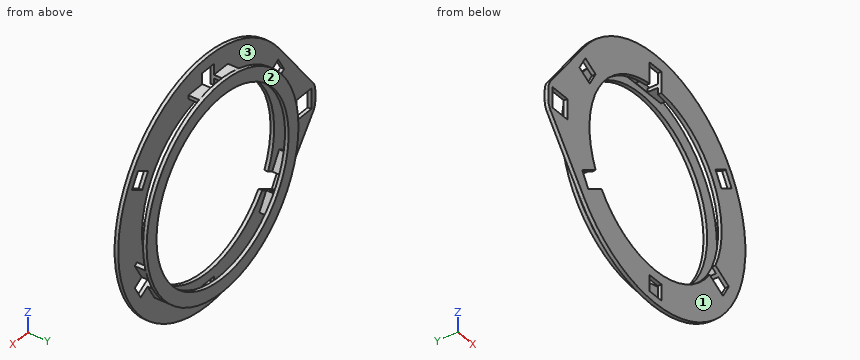
```python
from build123d import *

# Parameters (mm, degrees)
SKETCH1_R           = 340
SKETCH1_R_2         = 250
SKETCH1_W           = 44.45
SKETCH1_H           = 44.45
BOSS_EXTRUDE1_DEPTH = 10
BOSS_EXTRUDE2_DEPTH = 40
SKETCH3_W           = 44.45
SKETCH3_H           = 44.45
CUT_EXTRUDE1_DEPTH  = 30
CIRPATTERN1_COUNT   = 3
SKETCH4_R           = 287.263450512
SKETCH4_R_2         = 250
BOSS_EXTRUDE3_DEPTH = 10
BOSS_EXTRUDE4_DEPTH = 10
SKETCH6_W           = 57
SKETCH6_H           = 56.4
CUT_EXTRUDE2_DEPTH  = 10


with BuildPart() as part:
    # Sketch1 → Boss-Extrude1 (new body)
    with BuildSketch(Plane(origin=(0, 0, 0), x_dir=(1, 0, 0), z_dir=(0, 1, 0))):
        Circle(SKETCH1_R)
        Circle(SKETCH1_R_2, mode=Mode.SUBTRACT)
        with Locations((0, 297.225)):
            Rectangle(SKETCH1_W, SKETCH1_H, mode=Mode.SUBTRACT)
        Polygon((287.764315239, -140.477585401), (249.269486041, -118.252585401), (227.044486041, -156.747414599), (265.539315239, -178.972414599), align=None, mode=Mode.SUBTRACT)
        Polygon((-265.539315239, -178.972414599), (-227.044486041, -156.747414599), (-249.269486041, -118.252585401), (-287.764315239, -140.477585401), align=None, mode=Mode.SUBTRACT)
    extrude(amount=BOSS_EXTRUDE1_DEPTH)

    # Sketch2 → Boss-Extrude2 (add)
    with BuildSketch(Plane(origin=(0, 10, 0), x_dir=(1, 0, 0), z_dir=(0, 1, 0))):
        Polygon((22.25, -267.3), (-22.25, -267.3), (-75, -267.3), (-75, -277.3), (-22.25, -277.3), (22.25, -277.3), (75, -277.3), (75, -267.3), align=None)
        Polygon((-229.023844469, 157.919065234), (-202.648844469, 203.601905284), (-193.988590432, 198.601905284), (-220.363590432, 152.919065234), (-242.613590432, 114.380934766), (-268.988590432, 68.698094716), (-277.648844469, 73.698094716), (-251.273844469, 119.380934766), align=None)
        Polygon((251.273844469, 119.380934766), (277.648844469, 73.698094716), (268.988590432, 68.698094716), (242.613590432, 114.380934766), (220.363590432, 152.919065234), (193.988590432, 198.601905284), (202.648844469, 203.601905284), (229.023844469, 157.919065234), align=None)
    extrude(amount=BOSS_EXTRUDE2_DEPTH)

    # Sketch3 → Cut-Extrude1 (cut, symmetric)
    with BuildSketch(Plane.XY.offset(277.3)):
        with Locations((0, 16.699086593)):
            Rectangle(SKETCH3_W, SKETCH3_H)
    cut_extrude1 = extrude(amount=CUT_EXTRUDE1_DEPTH, both=True, mode=Mode.SUBTRACT)

    # CirPattern1: Cut-Extrude1 ×3 about axis
    cirpattern1_axis = Axis((0, 0, 0), (0, 1, 0))
    for i in range(1, CIRPATTERN1_COUNT):
        add(cut_extrude1.rotate(cirpattern1_axis, i * 360 / CIRPATTERN1_COUNT), mode=Mode.SUBTRACT)

    # Sketch4 → Boss-Extrude3 (add)
    with BuildSketch(Plane(origin=(0, 50, 0), x_dir=(1, 0, 0), z_dir=(0, 1, 0))):
        Circle(SKETCH4_R)
        Circle(SKETCH4_R_2, mode=Mode.SUBTRACT)
    extrude(amount=-BOSS_EXTRUDE3_DEPTH)

    # Sketch5 → Boss-Extrude4 (add)
    with BuildSketch(Plane(origin=(0, 0, 0), x_dir=(1, 0, 0), z_dir=(0, 1, 0))):
        with BuildLine():
            Line((-397.510704876, 39.376941903), (-270.390991444, 206.127901425))
            Line((-270.390991444, 206.127901425), (-330.879136225, 0))
            Line((-330.879136225, 0), (-270.390991444, -206.127901425))
            Line((-270.390991444, -206.127901425), (-397.510704876, -39.376941903))
            ThreePointArc((-397.510704876, -39.376941903), (-403.597415446, -27.924487201), (-405.7, -15.126600559))
            Line((-405.7, -15.126600559), (-405.7, 15.126600559))
            ThreePointArc((-405.7, 15.126600559), (-403.597415446, 27.924487201), (-397.510704876, 39.376941903))
        make_face()
        Polygon((-390.7, 0), (-390.7, 28.2), (-333.7, 28.2), (-333.7, -28.2), (-390.7, -28.2), align=None, mode=Mode.SUBTRACT)
    extrude(amount=BOSS_EXTRUDE4_DEPTH)

    # Sketch6 → Cut-Extrude2 (cut)
    with BuildSketch(Plane(origin=(0, 10, 0), x_dir=(-1, 0, 0), z_dir=(0, 1, 0))):
        with Locations((362.2, 0)):
            Rectangle(SKETCH6_W, SKETCH6_H)
    extrude(amount=-CUT_EXTRUDE2_DEPTH, mode=Mode.SUBTRACT)


solid = part.part
```
Can you work these out from the model? Positions are in its coordinate system, mm. Face numbers are marked on the shaded views. Give positions to 0.01 mm unless a question says otherwise; leave off trailing zeros. Order: outer loops, then holes, each group sorted by start corner. A loop starts at its lowest first (then second) coordinate and runs counter-clockwise, first axis right, second up. Notation, with made-up numbers: M 73.25,46 L 125.25,46 A16 cw 125.25,58 Z; hole C 14,1 d10. An arc over 180 degrees is marked long. Write item = value, one per line. Start each with the question number.
Q1. Suppose I cut it at D-D (z = 92.5). Write out the boundary of the cut face in (x, y).
Q2. Suppose I cut it at B-B (x = 0). Write out the boundary of the cut face in (y, z).
Q3. I need wall thicknesses on probe 1 along X at (y, z) = (42, 0); probe 2 along Y at (x, z) = (194, 194.5). Which ranges of each line are inside material? Lowest first, please. Write a range as [from, to].
Q4. Will these pins go through, and if not, where does the flat tip stop? pin 1 Ø3 at (y, z) = (43.5, -121.5) entering from -X; pin 2 Ø11 at (y, z) = (21, 270) entering from -X; pin 3 Ø5 at (x, y) = (-10, 6) entering from -Z.
Q5. Suppose I cut it at C-C (z = -90.5). Write out the boundary of the cut face in (x, y).
Q6. Suppose I cut it at A-A (z = 0). Write out the boundary of the cut face in (x, y), plus the area to 3 significant figures.
Q7. We'd pull the mould along Y, two halves only. Please class the marked faces 1, 2 and 3: pulls with the +Y half, pulls with the -Y half, needs draft (parallel to the pull), parting line crosses it, or undercut.
Check result:
q1.outline = M -357.01,0 L -232.26,0 L -232.26,10 L -357.01,10 Z; M -271.96,40 L -232.26,40 L -232.26,50 L -271.96,50 Z; M 232.26,0 L 327.18,0 L 327.18,10 L 232.26,10 Z; M 232.26,40 L 271.96,40 L 271.96,50 L 232.26,50 Z
q2.outline = M 0,-340 L 10,-340 L 10,-319.45 L 0,-319.45 Z; M 0,-275 L 10,-275 L 10,-250 L 0,-250 Z; M 0,307.3 L 10,307.3 L 10,340 L 0,340 Z; M 38.92,267.3 L 40,267.3 L 40,250 L 50,250 L 50,287.26 L 40,287.26 L 40,277.3 L 38.92,277.3 Z; M 40,-287.26 L 50,-287.26 L 50,-250 L 40,-250 Z
q3.probe_1 = [-287.26, -250], [250, 287.26]
q3.probe_2 = [0, 10], [40, 50]
q4.pin_1 = -261
q4.pin_2 = -75
q4.pin_3 = -339.92
q5.outline = M -358.54,0 L -233.04,0 L -233.04,10 L -256.4,10 L -256.4,40 L -233.04,40 L -233.04,50 L -272.64,50 L -272.64,40 L -267.95,40 L -267.95,10 L -358.54,10 Z; M 233.04,0 L 327.73,0 L 327.73,10 L 267.95,10 L 267.95,40 L 272.64,40 L 272.64,50 L 233.04,50 L 233.04,40 L 256.4,40 L 256.4,10 L 233.04,10 Z
q6.outline = M -405.7,0 L -390.7,0 L -390.7,10 L -405.7,10 Z; M -333.7,0 L -250,0 L -250,10 L -333.7,10 Z; M -287.26,40 L -250,40 L -250,50 L -287.26,50 Z; M 250,0 L 340,0 L 340,10 L 250,10 Z; M 250,40 L 287.26,40 L 287.26,50 L 250,50 Z
q6.area = 2,630 mm2
q7.face_1 = pulls with the -Y half
q7.face_2 = pulls with the +Y half
q7.face_3 = undercut
